Geometry: see drawing. Coordinates: mm, zero at the bounding-box minimum. A direction names the side the tool comes from. Coordinates: 2 decimals unless noted, no trailing zeros. Write each loop counter-clockwise with the first axis right and the second up, starting at its lowest first coordinate (ties: lowest second). Pieces come first, ordered by that corner, then holes. Notation, with made-up numbers: M 44,54.25 L 79,54.25 A18 ccw 79,61.25 Z; hole C 75,-28.75 d3. An arc over 180 degrees is marked long. Write item = value, one per line. Start each with the question number.
1. Access query for the marked faces 1 and 2. Directions: +Z, -Z, +X, -X, +Y, -Y. A direction counts if a zero-diameter tool reaches every point of the face in a straight line with its end or side. Return the directions, or none.
2. Line query: line 1 along Z through (x, y) = (5.5, 44); line 2 along X through (y, z) = (35, 14.5); line 3 along X through (y, z) = (41.5, 20.5) (1 decimal). Output: solid intervals per line, ascending.
3. Section query A-A (y = 14). Output: boundary loops of the cut face in (x, z).
4. Pin query (flat end, axial travel): pin 1 Ø1.5 at (x, y) = (11, 28) entering from -Z; pin 2 Ø15.5 at (y, z) = (25.5, 5) entering from -X. Return the tip coordinate at first contact, or that it passes through.
5. Section query B-B (x = 13.5). Output: boundary loops of the cut face in (y, z).
6. Section query C-C (z = 3). Output: boundary loops of the cut face in (x, y), then the cut area to 3 significant figures.
7. Pull-direction query (X, two-part tool) for the marked faces 3, 4 and 5; classes: pulls with the +X half, pulls with the -X half, needs draft (parallel to the pull), parting line crosses it, or undercut.
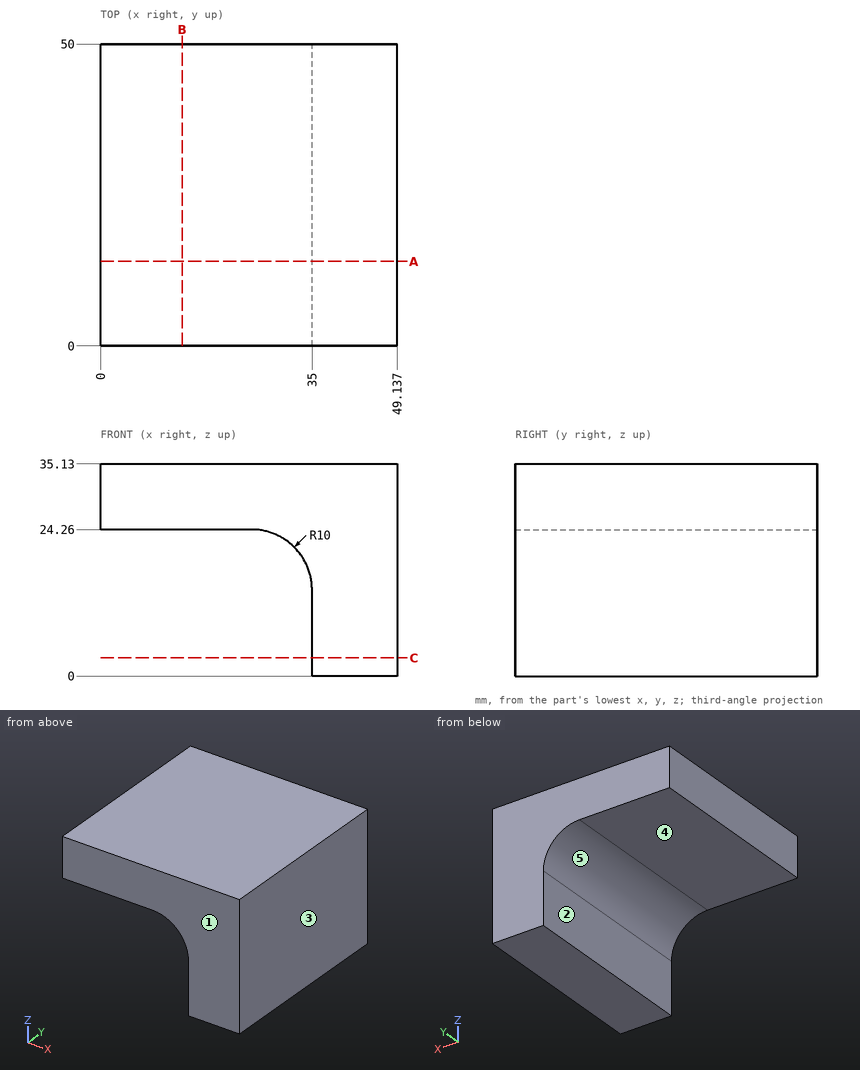
Results are:
q1.face_1 = +Z, -Z, +X, -X, -Y
q1.face_2 = -Z, -X, +Y, -Y
q2.line_1 = 24.26 to 35.13
q2.line_2 = 35 to 49.14
q2.line_3 = 32.8 to 49.1
q3.outline = M 0,24.26 L 25,24.26 A10 cw 35,14.26 L 35,0 L 49.14,0 L 49.14,35.13 L 0,35.13 Z
q4.pin_1 = 24.26
q4.pin_2 = 35
q5.outline = M 0,24.26 L 50,24.26 L 50,35.13 L 0,35.13 Z
q6.outline = M 35,0 L 49.14,0 L 49.14,50 L 35,50 Z
q6.area = 707 mm^2
q7.face_3 = pulls with the +X half
q7.face_4 = needs draft
q7.face_5 = pulls with the -X half
